```python
from build123d import *

# Parameters (mm, degrees)
SKETCH1_R            = 50
BOSS_EXTRUDE1_DEPTH  = 200
SKETCH2_R            = 10
BOSS_EXTRUDE2_DEPTH  = 5
FILLET1_R            = 1
FILLET1_OF_MIRROR3_R = 1


with BuildPart() as part:
    # Sketch1 → Boss-Extrude1 (new, symmetric)
    with BuildSketch(Plane(origin=(0, 0, 0), x_dir=(0, 0, -1), z_dir=(1, 0, 0))):
        Circle(SKETCH1_R)
    extrude(amount=BOSS_EXTRUDE1_DEPTH, both=True)

    # Sketch2 → Boss-Extrude2 (add)
    with BuildSketch(Plane(origin=(200, 0, 0), x_dir=(0, 0, -1), z_dir=(1, 0, 0))):
        Circle(SKETCH2_R)
    boss_extrude2 = extrude(amount=BOSS_EXTRUDE2_DEPTH)

    # Fillet1
    fillet1_edges = [part.edges().sort_by_distance(p)[0] for p in [
        (205, 0, 10),
    ]]
    fillet(fillet1_edges, radius=FILLET1_R)

    # Mirror3: Boss-Extrude2 across plane
    add(boss_extrude2.mirror(Plane(origin=(0, 0, 0), x_dir=(0, 0, 1), z_dir=(1, 0, 0))))

    # Fillet1 of Mirror3
    fillet1_of_mirror3_edges = [part.edges().sort_by_distance(p)[0] for p in [
        (-205, 0, 10),
    ]]
    fillet(fillet1_of_mirror3_edges, radius=FILLET1_OF_MIRROR3_R)


solid = part.part
```
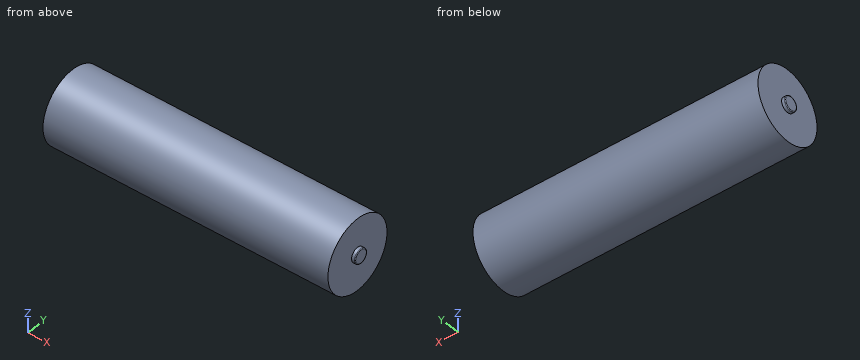
Geometry: final body of the model. Coordinates: model frame, mm. Round coordinates to 2 decimals unless told otherwise and drop trailing zeros. Order: outer loops, then holes, each group sorted by start corner. A loop starts at its lowest first (then second) coordinate and runs counter-clockwise, first axis right, second up. Notation, with made-up numbers: M 18.25,33.5 L 45.25,33.5 A27 cw 45.25,56.5 Z; hole C 60.5,-13 d9. An arc over 180 degrees is marked long. Use one line per item in the form item = value. Start each with the question number.
Q1. Pin query (flat end, axial travel): pin 1 Ø12 at (x, y) = (-111.5, -23.5) entering from +Z; pin 2 Ø10 at (x, z) = (-109, -6.5) entering from -Y; pin 3 Ø2 at (x, y) = (9.5, 7) entering from -Z. Return the tip coordinate at first contact, or that it passes through.
Q2. Cut plane C-C (x = -85.5). Return loops of the section in (y, z).
Q3. Material intervals for line 1 (Y direction, x = 64, z = 1.5); line 2 (X direction, y = 4, z = -31), sorted ascending. Write a range as [from, to].
Q4. Cut plane A-A (z = 0). Return loops of the section in (x, y), and give its area (3 significant figures).
Q5. Cut plane D-D (z = 29.5). Return loops of the section in (x, y).
Geometry results:
q1.pin_1 = 46.84
q1.pin_2 = -49.98
q1.pin_3 = -49.64
q2.outline = C 0,0 d100
q3.line_1 = [-49.98, 49.98]
q3.line_2 = [-200, 200]
q4.outline = M -205,-9 A1 ccw -204,-10 L -200,-10 L -200,-50 L 200,-50 L 200,-10 L 204,-10 A1 ccw 205,-9 L 205,9 A1 ccw 204,10 L 200,10 L 200,50 L -200,50 L -200,10 L -204,10 A1 ccw -205,9 Z
q4.area = 40,200 mm^2
q5.outline = M -200,-40.37 L 200,-40.37 L 200,40.37 L -200,40.37 Z
